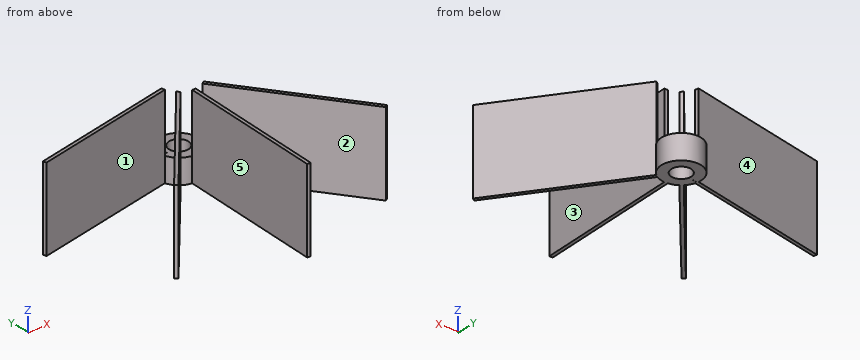
from build123d import *

# Parameters (mm, degrees)
BOSS_EXTRUDE2_DEPTH = 25
BOSS_EXTRUDE3_DEPTH = 60


with BuildPart() as part:
    # Sketch1 → Boss-Extrude2 (new body)
    with BuildSketch(Plane.XY):
        with BuildLine():
            ThreePointArc((-19.272609064, -5.344767522), (-17.431181917, -9.805809349), (-14.574748022, -13.695865072))
            Line((-14.574748022, -13.695865072), (-114.51684862, -125.551023774))
            Line((-114.51684862, -125.551023774), (-111.917163437, -127.873831243))
            Line((-111.917163437, -127.873831243), (-11.975062839, -16.018672542))
            ThreePointArc((-11.975062839, -16.018672542), (-7.744084669, -18.43987941), (-3.053041676, -19.765599827))
            Line((-3.053041676, -19.765599827), (-12.943579656, -169.439168831))
            Line((-12.943579656, -169.439168831), (-9.464936702, -169.66904008))
            Line((-9.464936702, -169.66904008), (0.425601277, -19.995471076))
            ThreePointArc((0.425601277, -19.995471076), (5.250301367, -19.298557862), (9.763088678, -17.455145358))
            Line((9.763088678, -17.455145358), (94.117488701, -141.488750468))
            Line((94.117488701, -141.488750468), (97.000219629, -139.528225031))
            Line((97.000219629, -139.528225031), (12.645819606, -15.494619921))
            ThreePointArc((12.645819606, -15.494619921), (7.698899748, 18.45879039), (-19.907923967, -1.91691505))
            Line((-19.907923967, -1.91691505), (-167.528286005, -28.529481853))
            Line((-167.528286005, -28.529481853), (-166.892971102, -31.957334324))
            Line((-166.892971102, -31.957334324), (-19.272609064, -5.344767522))
        make_face()
        with BuildLine():
            Line((-19.682714938, -3.54834224), (-9.841357469, -1.77417112))
            ThreePointArc((-9.841357469, -1.77417112), (9.836982775, 1.798268581), (-9.832549076, -1.822355255))
            Line((-9.832549076, -1.822355255), (-19.665098151, -3.64471051))
            ThreePointArc((-19.665098151, -3.64471051), (-19.67396555, -3.596537162), (-19.682714938, -3.54834224))
        make_face(mode=Mode.SUBTRACT)
    extrude(amount=BOSS_EXTRUDE2_DEPTH)

    # Sketch2 → Boss-Extrude3 (add)
    with BuildSketch(Plane.XY.offset(25)):
        Polygon((-167.528286005, -28.529481853), (-166.892971102, -31.957334324), (-19.272609064, -5.344767522), (-19.907923967, -1.91691505), align=None)
        Polygon((-14.574748022, -13.695865072), (-11.975062839, -16.018672542), (-111.917163437, -127.873831243), (-114.51684862, -125.551023774), align=None)
        Polygon((-3.053041676, -19.765599827), (0.425601277, -19.995471076), (-9.464936702, -169.66904008), (-12.943579656, -169.439168831), align=None)
        Polygon((9.763088678, -17.455145358), (12.645819606, -15.494619921), (97.000219629, -139.528225031), (94.117488701, -141.488750468), align=None)
    extrude(amount=BOSS_EXTRUDE3_DEPTH)


solid = part.part
For this review, take the finished solid that the model builds, in its own axes (mm). Face numbers are marked on the shaded views. A direction names the side the tool comes from. Round coordinates to 2 decimals unless told otherwise and drop trailing zeros. Order: outer loops, then holes, each group sorted by start corner. A loop starts at its lowest first (then second) coordinate and runs counter-clockwise, first axis right, second up. Notation, with made-up numbers: M 83.25,-32 L 119.25,-32 A33 cw 119.25,2 Z; hole C 53,64.25 d1. An arc over 180 degrees is marked long. Write each question's results on one line, items separated by ' | '. Start each with the question number.
1. Add section B-B (x = 17). State the section outline as (y, z) points.
2. Tool access review of the marked faces 1 and 2: name each direction out of +Z, -Z, +X, -X, +Y, -Y from which nothing blocks a thin tool from reaching the whole face with its end or side.
3. To check wall thickness, follow L1, parallel to X at y = 0, z = 13; L2, parallel to X at y = -84, z = 35.5; L3, parallel to X at y = -32, z = 79.5. State the ranges of each line that lie inside material, in increasing order. Write a range as [from, to].
4. Draft analysis for pull direction Y (two halves, no side actions). For the marked faces 3, 4 and 5, state which applies: pulls with the +Y half, pulls with the -Y half, needs draft (parallel to the pull), parting line crosses it, or undercut.
5. Add section D-D (y = -102.5). State the section outline as (x, z) points, then the cut area to 3 significant figures.
6. Add section C-C (z = 48.5). State the section outline as (x, y) points.
7. Clearance check with flat-ended pins moving along their axes: pin 1 Ø10 at (x, z) = (-12, 23) entering from -Y; pin 2 Ø4 at (y, z) = (-29, 50.5) entering from +X; pin 3 Ø2 at (y, z) = (-137, 14.5) entering from +X; pin 4 Ø4 at (x, z) = (-133, 48) entering from +Y. State where each tip first meets the part, or that it passes through.
8. Add section A-A (z = 13.5). State the section outline as (x, y) points.
Output values:
1) outline: M -28.1,0 L -21.9,0 L -21.9,85 L -28.1,85 Z; M -10.54,0 L 10.54,0 L 10.54,25 L -10.54,25 Z
2) face 1: +Z, -Z | face 2: +Z, -Z, -Y
3) L1: [-20, -10], [10, 20] | L2: [-77.39, -72.72], [-7.3, -3.8], [55.02, 59.24] | L3: [-30.93, -26.25], [-3.86, -0.37], [19.65, 23.87]
4) face 3: pulls with the -Y half | face 4: pulls with the +Y half | face 5: undercut
5) outline: M -93.92,0 L -89.25,0 L -89.25,85 L -93.92,85 Z; M -8.52,0 L -5.03,0 L -5.03,85 L -8.52,85 Z; M 67.6,0 L 71.82,0 L 71.82,85 L 67.6,85 Z | area: 1,050 mm^2
6) outline: M -167.53,-28.53 L -166.89,-31.96 L -19.27,-5.34 L -19.91,-1.92 Z; M -114.52,-125.55 L -111.92,-127.87 L -11.98,-16.02 L -14.57,-13.7 Z; M -12.94,-169.44 L -9.46,-169.67 L 0.43,-20 L -3.05,-19.77 Z; M 9.76,-17.46 L 94.12,-141.49 L 97,-139.53 L 12.65,-15.49 Z
7) pin 1: y = -169.67 | pin 2: x = 23.19 | pin 3: x = 95.96 | pin 4: y = -21.94
8) outline: M -167.53,-28.53 L -166.89,-31.96 L -19.27,-5.34 A20 ccw -14.57,-13.7 L -114.52,-125.55 L -111.92,-127.87 L -11.98,-16.02 A20 ccw -3.05,-19.77 L -12.94,-169.44 L -9.46,-169.67 L 0.43,-20 A20 ccw 9.76,-17.46 L 94.12,-141.49 L 97,-139.53 L 12.65,-15.49 A20 ccw long -19.91,-1.92 Z; hole M -19.68,-3.55 A20 ccw -19.67,-3.64 L -9.83,-1.82 A10 ccw long -9.84,-1.77 Z
